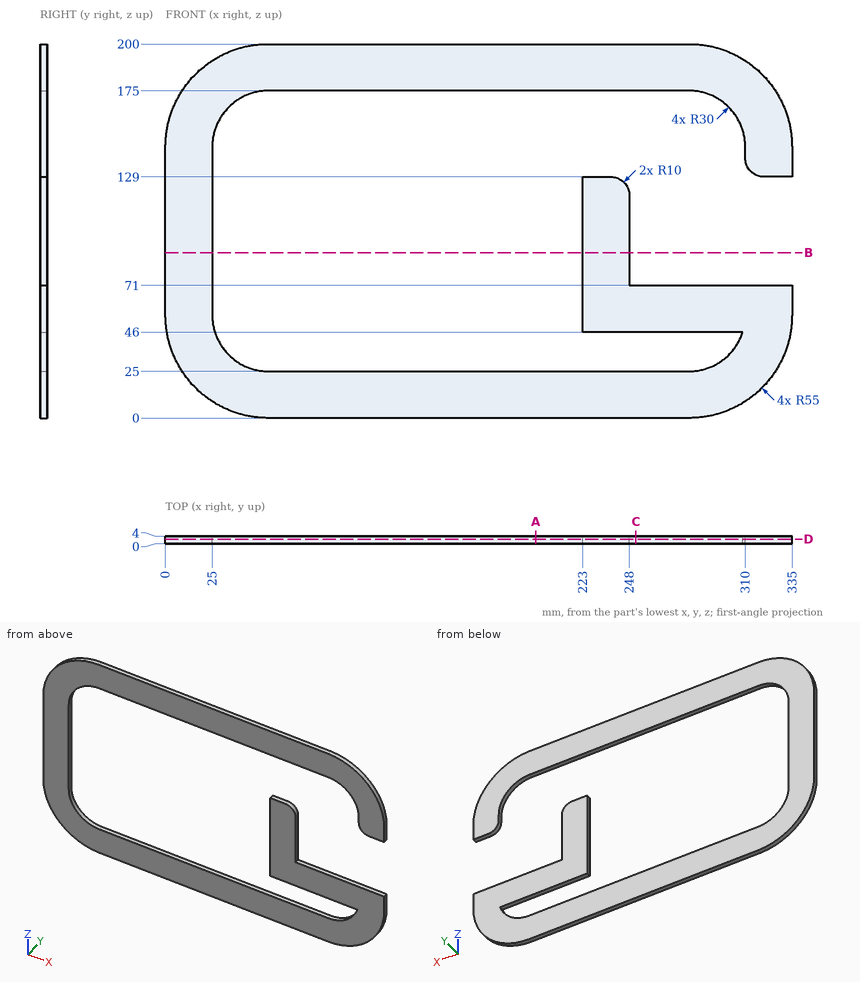
Source: three-view drawing plus pictorial views. Frame: mm from the lowest corner of the part. Coordinates: 2 decimals unless noted, no trailing zeros. Write each loop counter-clockwise with the first axis right and the second up, starting at its lowest first coordinate (ties: lowest second). Pieces come first, ordered by that corner, then holes. Notation, with made-up numbers: (4.25, 33) -> (43.25, 33) arc R24 ccw to (43.25, 62) -> close; hole circle Ø2 at (-2.75, 76). An arc over 180 degrees is marked (long way). Write each question's results on one line, items separated by ' | '.
Item 1: Section query D-D on y = 2.3. Return loops of the section in (x, z).
Conclusion:
outline: (0, 55) arc R55 ccw to (55, 0) -> (280, 0) arc R55 ccw to (335, 55) -> (335, 71) -> (248, 71) -> (248, 119) arc R10 ccw to (238, 129) -> (223, 129) -> (223, 46) -> (308.62, 46) arc R30 cw to (280, 25) -> (55, 25) arc R30 cw to (25, 55) -> (25, 145) arc R30 cw to (55, 175) -> (280, 175) arc R30 cw to (310, 145) -> (310, 139) arc R10 ccw to (320, 129) -> (335, 129) -> (335, 145) arc R55 ccw to (280, 200) -> (55, 200) arc R55 ccw to (0, 145) -> close
Item 2: Section query A-A on x = 198. Return loops of the section in (y, z).
Conclusion:
outline: (0, 0) -> (4, 0) -> (4, 25) -> (0, 25) -> close; (0, 175) -> (4, 175) -> (4, 200) -> (0, 200) -> close
Item 3: Section query C-C on x = 251.5. Return loops of the section in (y, z), plus the area to 3 significant figures.
Conclusion:
outline: (0, 0) -> (4, 0) -> (4, 25) -> (0, 25) -> close; (0, 46) -> (4, 46) -> (4, 71) -> (0, 71) -> close; (0, 175) -> (4, 175) -> (4, 200) -> (0, 200) -> close | area: 300 mm^2
Item 4: Material intervals for probe 1 along Z at (x, y) = (237, 3.5); probe 2 along Z at (x, y) = (116.5, 2.15); probe 3 along Z at (x, y) = (273, 2), sorted ascending.
Conclusion:
probe 1: z = 0 to 25, 46 to 129, 175 to 200 | probe 2: z = 0 to 25, 175 to 200 | probe 3: z = 0 to 25, 46 to 71, 175 to 200
Item 5: Pin query (flat end, axial travel): pin 1 Ø1.2 at (y, z) = (2, 99) entering from +X; pin 2 Ø2 at (y, z) = (3.5, 162.5) entering from -X; pin 3 Ø1.5 at (y, z) = (1.5, 157) entering from -X. Return the tip coordinate at first contact, or that it passes through.
Conclusion:
pin 1: stops at x = 248 | pin 2: stops at x = 2.53 | pin 3: stops at x = 1.16
Item 6: Section query B-B on z = 88.5. Return loops of the section in (x, y), plus the area to 3 significant figures.
Conclusion:
outline: (0, 0) -> (25, 0) -> (25, 4) -> (0, 4) -> close; (223, 0) -> (248, 0) -> (248, 4) -> (223, 4) -> close | area: 200 mm^2
